```python
from build123d import *

# Parameters (mm, degrees)
SKETCH1_R           = 0.5
BOSS_EXTRUDE1_DEPTH = 15.5
SKETCH1_3_R         = 1.2
SKETCH1_3_R_2       = 0.5
BOSS_EXTRUDE2_DEPTH = 4.75
FILLET1_R           = 0.2
SKETCH2_R           = 0.85
BOSS_EXTRUDE3_DEPTH = 0.3
SKETCH4_W           = 0.465575533
SKETCH4_H           = 0.034477487
SKETCH5_W           = 1.257485092
SKETCH5_H           = 2.46
SKETCH6_R           = 0.5
BOSS_EXTRUDE4_DEPTH = 2.84


with BuildPart() as part:
    # Sketch1 → Boss-Extrude1 (new body)
    with BuildSketch(Plane.XY):
        Circle(SKETCH1_R)
    extrude(amount=BOSS_EXTRUDE1_DEPTH)



with BuildPart() as body_2:
    # Sketch1<3> → Boss-Extrude2 (new body)
    with BuildSketch(Plane.XY):
        Circle(SKETCH1_3_R)
        Circle(SKETCH1_3_R_2, mode=Mode.SUBTRACT)
    extrude(amount=-BOSS_EXTRUDE2_DEPTH)

    # Fillet1
    fillet1_edges = [body_2.edges().sort_by_distance(p)[0] for p in [
        (-1.2, 0, 0),
    ]]
    fillet(fillet1_edges, radius=FILLET1_R)


with BuildPart() as part_1:
    add(part.part)

    add(body_2.part)  # Boss-Extrude3 merges body 2
    # Sketch2 → Boss-Extrude3 (add)
    with BuildSketch(Plane.XY):
        Circle(SKETCH2_R)
    extrude(amount=BOSS_EXTRUDE3_DEPTH)

    # Sketch3 → Revolve1 (revolve)
    with BuildSketch(Plane(origin=(0, 0, 0), x_dir=(1, 0, 0), z_dir=(0, 1, 0))):
        with BuildLine():
            Line((0.5, -15.5), (0, -15.5))
            Line((0, -15.5), (0, -16.0775))
            ThreePointArc((0, -16.0775), (0.247487373, -16.180012627), (0.35, -16.4275))
            Line((0.35, -16.4275), (0.5, -16.4275))
            ThreePointArc((0.5, -16.4275), (0.472905202, -16.265140307), (0.39455732, -16.120377026))
            Line((0.39455732, -16.120377026), (0.39455732, -16.001977042))
            Line((0.39455732, -16.001977042), (0.513344718, -16.001977042))
            Line((0.513344718, -16.001977042), (0.513344718, -15.7758978))
            Line((0.513344718, -15.7758978), (0.386893617, -15.7758978))
            ThreePointArc((0.386893617, -15.7758978), (0.416267844, -15.626806679), (0.5, -15.5))
        make_face()
    revolve(axis=Axis((0, 0, 15.5), (0, 0, 1)))

    # Sketch4 → Revolve2 (revolve)
    with BuildSketch(Plane(origin=(0, 0, 0), x_dir=(1, 0, 0), z_dir=(0, 1, 0))):
        with Locations((-0.232787767, -16.322761257)):
            Rectangle(SKETCH4_W, SKETCH4_H)
    revolve(axis=Axis((0, 0, 16.305522513), (0, 0, 1)))

    # Sketch5 → Cut-Revolve1 (revolve, cut)
    with BuildSketch(Plane(origin=(0, 0, 0), x_dir=(1, 0, 0), z_dir=(0, 1, 0))):
        with Locations((-0.924942546, -14.27)):
            Rectangle(SKETCH5_W, SKETCH5_H)
    revolve(axis=Axis((0, 0, 15.5), (0, 0, 1)), mode=Mode.SUBTRACT)

    # Sketch6 → Boss-Extrude4 (add)
    with BuildSketch(Plane(origin=(0, 0, -4.75), x_dir=(-1, 0, 0), z_dir=(0, 0, -1))):
        Circle(SKETCH6_R)
    extrude(amount=-BOSS_EXTRUDE4_DEPTH)


solid = part_1.part
```
Build history of the part. All positions in model axes, mm. Give positions to 0.01 mm unless a question says otherwise; leave off trailing zeros. Loops run counter-clockwise (first coordinate to the right, second up) from the corner with the lowest first, then second, coordinate; pieces in that order, holes last.
Item 1: Slice it at B-B, the plane y = 0. Give the number of separate pieces and of enclosed holes in the cut face, and give its area (3 significant figures).
Answers follow:
separate pieces: 1
enclosed holes: 2
area: 24.9 mm2
Item 2: Slice it at A-A, the plane z = 14.5. List the corners of the cut face in (x, y).
Answers follow:
outline: circle Ø0.59 at (0, 0)
Item 3: Pull direction Z, two halves, no side cores. Call faces 1 (the face through (0.65, 1.01, -2.44)), 2 (the face through (0, 0, 0)), 3 (the face through (0, 0, -4.75)): released by +Z, released by -Z, zero draft, split by the parting line, or undercut.
Answers follow:
face 1: zero draft
face 2: undercut
face 3: released by -Z
Item 4: Drill centre lines: line 1 (Y direction, x = 0, z = -1.5); line 2 (Z direction, x = 0.8, y = -0.45); line 3 (Y direction, x = 0.4, z = 8). Where is each one in solid material? Low to high.
Answers follow:
line 1: y = -1.2 to -0.5, 0.5 to 1.2
line 2: z = -4.75 to 0
line 3: y = -0.3 to 0.3
Item 5: Flat gauge pin, fed straight in: pin 1 (0.5 mm diameter, centred on x = 0, y = 0, fed in from +Z). Where does the tip first touch, or does it go through?
Answers follow:
pin 1: stops at z = 16.34
Item 6: Slice it at D-D, the plane z = -3. List the corners of the cut face in (x, y).
Answers follow:
outline: circle Ø2.4 at (0, 0)
